```python
from build123d import *

# Parameters (mm, degrees)
F0_R     = 4
F2_DEPTH = 6.5
F0_R_2   = 2
F3_DEPTH = 6
F5_D     = 3.3
F5_DEPTH = 15
F5_TIP   = 0.9914200214


with BuildPart() as f2:
    # F0 (on Top) → F2 (new body)
    with BuildSketch(Plane.XY):
        with BuildLine():
            ThreePointArc((-5.5, 0), (0, -5.5), (5.5, 0))
            ThreePointArc((5.5, 0), (5.4755595256, 0.5179265218), (5.4024553156, 1.03125))
            ThreePointArc((5.4024553156, 1.03125), (0, 5.5), (-5.4024553156, 1.03125))
            ThreePointArc((-5.4024553156, 1.03125), (-5.4755595256, 0.5179265218), (-5.5, 0))
        make_face()
        Circle(F0_R, mode=Mode.SUBTRACT)
    extrude(amount=F2_DEPTH)

    # F0 (on Top) → F3 (join)
    with BuildSketch(Plane.XY):
        with BuildLine():
            ThreePointArc((-5.4024553156, 1.03125), (0, 5.5), (5.4024553156, 1.03125))
            Line((5.4024553156, 1.03125), (3.9290584114, 8.75))
            ThreePointArc((3.9290584114, 8.75), (0, 12), (-3.9290584114, 8.75))
            Line((-3.9290584114, 8.75), (-5.4024553156, 1.03125))
        make_face()
        with Locations((0, 8)):
            Circle(F0_R_2, mode=Mode.SUBTRACT)
        with BuildLine():
            Line((14.4568322948, -4), (5.5, 0))
            ThreePointArc((5.5, 0), (0, -5.5), (-5.5, 0))
            Line((-5.5, 0), (-14.4568322948, -4))
            ThreePointArc((-14.4568322948, -4), (0, -15), (14.4568322948, -4))
        make_face()
    extrude(amount=F3_DEPTH)

    # F5
    with Locations(Plane.XZ.offset(15)):
        with Locations((0, 3)):
            Hole(F5_D / 2, depth=F5_DEPTH)
            with Locations((0, 0, -(F5_DEPTH + F5_TIP / 2))):  # 118° drill point
                Cone(0, F5_D / 2, F5_TIP, mode=Mode.SUBTRACT)


solid = f2.part
```
Design review of the part built by this model. Coordinates are the model's own, in mm. A direction names the side the tool comes from. Coordinates: 2 decimals unless noted, no trailing zeros. Loops run counter-clockwise (first coordinate to the right, second up) from the corner with the lowest first, then second, coordinate; pieces in that order, holes last.
Q1. To check wall thickness, follow line 1 (Y direction, x = 0, z = 4.75); line 2 (Y direction, x = 0, z = 2.75); line 3 (Z direction, x = 0, y = -5.75). State the ranges of each line that lie inside material, in increasing order.
Reported:
line 1: y = -15 to -4, 4 to 6, 10 to 12
line 2: y = 4 to 6, 10 to 12
line 3: z = 0 to 1.35, 4.65 to 6
Q2. We need section B-B on x = -3. State the section outline as (y, z) points, and give its area (3 significant figures).
Reported:
outline: (-14.7, 0) - (-2.65, 0) - (-2.65, 6.5) - (-4.61, 6.5) - (-4.61, 6) - (-14.7, 6) - close; (2.65, 0) - (10.65, 0) - (10.65, 6) - (4.61, 6) - (4.61, 6.5) - (2.65, 6.5) - close
area: 122 mm2
Q3. For pin 1 (9 mm diameter, centred on x = 0, y = 0, fed in from -Z); pin 2 (3 mm diameter, centred on y = 6, z = 2, fed in from -X), all flat-tipped, find the tip position at first contact; note any pin that passes through.
Reported:
pin 1: stops at z = 0
pin 2: stops at x = -4.74
Q4. We need section D-D on x = 4.75. State the section outline as (y, z) points, and give its area (3 significant figures).
Reported:
outline: (-14.23, 0) - (4.45, 0) - (4.45, 6) - (2.77, 6) - (2.77, 6.5) - (-2.77, 6.5) - (-2.77, 6) - (-14.23, 6) - close
area: 115 mm2
Q5. We need section A-A on x = 0. State the section outline as (y, z) points.
Reported:
outline: (-15, 0) - (-4, 0) - (-4, 1.35) - (-15, 1.35) - close; (-15, 4.65) - (-4, 4.65) - (-4, 6.5) - (-5.5, 6.5) - (-5.5, 6) - (-15, 6) - close; (4, 0) - (6, 0) - (6, 6) - (5.5, 6) - (5.5, 6.5) - (4, 6.5) - close; (10, 0) - (12, 0) - (12, 6) - (10, 6) - close
Q6. We need section C-C on y = -4.75. State the section outline as (x, z) points, and give its area (3 significant figures).
Reported:
outline: (-14.23, 0) - (14.23, 0) - (14.23, 6) - (2.77, 6) - (2.77, 6.5) - (-2.77, 6.5) - (-2.77, 6) - (-14.23, 6) - close; hole circle Ø3.3 at (0, 3)
area: 165 mm2
Q7. The part is to be moulded in two halves that separate along X. For faces 3 (the face through (-4, -2, 6.5)), 4 (the face through (0, -15, 1)), 5 (the face through (-4.655, 4.945, 2.958)), 6 (the face through (2.15, 3.373, 3.204)), say which applies: +X half, -X half, draft (parallel to the pull), parting line (faces both ways), or undercut.
Reported:
face 3: draft
face 4: parting line
face 5: -X half
face 6: undercut
Q8. Tool access review of faces 1 (the face through (0.215, -9.244, 4.636)), 2 (the face through (0, 12, 3)): name each direction out of +Z, -Z, +X, -X, +Y, -Y from which nothing blocks a thin tool from reaching the whole face with its end or side.
Reported:
face 1: -Y
face 2: +Z, -Z, +Y
